Can you work these out from the model? Positions are in its coordinate system, mm. Round coordinates to 2 decimals unless told otherwise and drop trailing zeros. Loops run counter-clockwise (first coordinate to the right, second up) from the corner with the lowest first, then second, coordinate; pieces in that order, holes last.
(1) Will this pin go through, and if not, where does the flat tip stop? pin 1 Ø4 at (x, z) = (13, -52) entering from -Y.
(2) I want a section at B-B on x = -31. Write out the boundary of the cut face in (y, z).
(3) If I drill on line 1 along Z through (x, y) = (13, 0.7) (3 decimals); line 2 along X through (y, z) = (1, -52) (3 decimals); line 3 along X through (y, z) = (0.8, -125), over which ranges is the centre line in solid material (lowest first)?
(4) I want a section at A-A on z = -161.5. Write out the boundary of the cut face in (x, y), plus the area to 3 significant figures.
(5) I want a section at D-D on x = 13. Write out the boundary of the cut face in (y, z) (3 decimals), plus the area to 3 significant figures.
(6) Thinking about a two-plate mould opening in X: for faces 1 (the face through (12.59, 1.52, -191.15)), 2 (the face through (12.31, 1.52, -48.9)), 3 (the face through (-189, 3, -118)), which applies, released by +X, released by -X, zero draft, split by the parting line, or undercut?
(7) I want a section at C-C on y = 0.5. Write out the boundary of the cut face in (x, z) (3 decimals).
Autodesk Inventor part; units mm, degrees
ref_plane "YZ Plane" through (0, 0, 0) normal (1, 0, 0) x (0, 1, 0)
ref_plane "XZ Plane" through (0, 0, 0) normal (0, 1, 0) x (-1, 0, 0)
ref_plane "XY Plane" through (0, 0, 0) normal (0, 0, 1) x (1, 0, 0)
sketch "Boceto1" plane through (0, 0, 0) normal (0, 1, 0) x (-1, 0, 0)
  line L0 (0, 0) -> (180, 0)
  line L1 (180, 0) -> (180, -240)
  line L2 (180, -240) -> (0, -240)
  line L3 (0, -240) -> (0, 0)
  line L4 (-3, -243) -> (183, -243)
  line L5 (183, -243) -> (183, 3)
  line L6 (183, 3) -> (-3, 3)
  line L7 (-3, 3) -> (-3, -243)
  line L8 (203, 23) -> (203, -263)
  line L9 (203, -263) -> (-23, -263)
  line L10 (-23, -263) -> (-23, 23)
  line L11 (-23, 23) -> (203, 23)
  dimension "d0" = 180
  dimension "d1" = 240
  dimension "d2" = 3
  dimension "d5" = 20
extrude "Extrusión3" add sketch "Boceto1" along normal blind 3 contours L8 L9 L10 L11
sketch "Boceto6" plane through (0, 3, 0) normal (0, 1, 0) x (1, 0, 0)
  line L0 (-183, -3) -> (-183, 243)
  line L1 (-183, 243) -> (3, 243)
  line L2 (3, 243) -> (3, -3)
  line L3 (3, -3) -> (-183, -3)
  line L4 (-203, 263) -> (-203, -23)
  line L5 (-203, -23) -> (23, -23)
  line L6 (23, -23) -> (23, 263)
  line L7 (23, 263) -> (-203, 263)
  line L8 (23, 91.3088) -> (23, 114.6899)
  line L9 (3, 114.6899) -> (3, 91.3088)
  circle A0 centre (13, 188) radius 3.175
  circle A1 centre (13, 52) radius 3.175
  point P0 (0, 0)
  dimension "d32" = 6.35
  dimension "d33" = 75
  dimension "d34" = 6.35
  dimension "d35" = 75
extrude "Extrusión8" cut sketch "Boceto6" against normal blind 3 contours A0 | A1
properties part number "Tapa Superior"
Filled sheet:
1. pin 1: passes through
2. outline: (0, -263) - (3, -263) - (3, -243) - (0, -243) - close; (0, 3) - (3, 3) - (3, 23) - (0, 23) - close
3. line 1: z = -263 to -191.175, -184.825 to -55.175, -48.825 to 23
3. line 2: x = -203 to -183, 3 to 9.825, 16.175 to 23
3. line 3: x = -203 to -183, 3 to 23
4. outline: (-203, 0) - (-183, 0) - (-183, 3) - (-203, 3) - close; (3, 0) - (23, 0) - (23, 3) - (3, 3) - close
4. area: 120 mm2
5. outline: (0, -263) - (3, -263) - (3, -191.175) - (0, -191.175) - close; (0, -184.825) - (3, -184.825) - (3, -55.175) - (0, -55.175) - close; (0, -48.825) - (3, -48.825) - (3, 23) - (0, 23) - close
5. area: 820 mm2
6. face 1: undercut
6. face 2: undercut
6. face 3: zero draft
7. outline: (-203, -263) - (23, -263) - (23, 23) - (-203, 23) - close; hole (-183, -243) - (3, -243) - (3, 3) - (-183, 3) - close; hole circle Ø6.35 at (13, -188); hole circle Ø6.35 at (13, -52)
